```python
from build123d import *

# Parameters (mm, degrees)
SKETCH_1_R          = 20
SKETCH_1_R_2        = 1.6
EXTRUDE_1_DEPTH     = 2.5
SWEEP_1_PROFILE_R   = 5
EXTRUDE_2_DEPTH     = 2.5
SKETCH_10_W         = 23
SKETCH_10_H         = 44.650800955
CUT_EXTRUDE_1_DEPTH = 2
SKETCH_11_R         = 2.5
CUT_EXTRUDE_2_DEPTH = 21.5
FILLET_1_R          = 5


with BuildPart() as part:
    # 草图1 → 凸台-拉伸1 (new body, symmetric)
    with BuildSketch(Plane.XY):
        Circle(SKETCH_1_R)
        with Locations((0, 15)):
            Circle(SKETCH_1_R_2, mode=Mode.SUBTRACT)
        with Locations((15, 0)):
            Circle(SKETCH_1_R_2, mode=Mode.SUBTRACT)
        with Locations((0, -15)):
            Circle(SKETCH_1_R_2, mode=Mode.SUBTRACT)
        with Locations((-15, 0)):
            Circle(SKETCH_1_R_2, mode=Mode.SUBTRACT)
    extrude(amount=EXTRUDE_1_DEPTH, both=True)

    # 扫描1: sweep along a path in 草图4
    with BuildLine(Plane(origin=(0, 0, 0), x_dir=(1, 0, 0), z_dir=(0, 1, 0))) as sweep_1_path:
        Line((0, 0), (0, 60))
    # 扫描1 profile (on start of the path) → 扫描1 (sweep)
    with BuildSketch(Plane(origin=(0, 0, 0), x_dir=(-1, 0, 0), z_dir=(0, 0, -1))):
        Circle(SWEEP_1_PROFILE_R)
    sweep(path=sweep_1_path.line)

    # 草图9 → 凸台-拉伸2 (add, symmetric)
    with BuildSketch(Plane(origin=(0, 0, 0), x_dir=(1, 0, 0), z_dir=(0, 1, 0))):
        with BuildLine():
            Line((13.5, 90), (13.5, 60))
            ThreePointArc((13.5, 60), (0, 46.5), (-13.5, 60))
            Line((-13.5, 60), (-13.5, 90))
            ThreePointArc((-13.5, 90), (0, 103.5), (13.5, 90))
        make_face()
    extrude(amount=EXTRUDE_2_DEPTH, both=True)

    # 草图10 → 切除-拉伸1 (cut)
    with BuildSketch(Plane(origin=(0, 2.5, 0), x_dir=(1, 0, 0), z_dir=(0, 1, 0))):
        with Locations((0, 82.325400478)):
            Rectangle(SKETCH_10_W, SKETCH_10_H)
    extrude(amount=-CUT_EXTRUDE_1_DEPTH, mode=Mode.SUBTRACT)

    # 草图11 → 切除-拉伸2 (cut, through all)
    with BuildSketch(Plane(origin=(0, 0.5, 0), x_dir=(1, 0, 0), z_dir=(0, 1, 0))):
        with Locations((-6.75, 64)):
            Circle(SKETCH_11_R)
        with Locations((6.75, 64)):
            Circle(SKETCH_11_R)
    extrude(amount=-CUT_EXTRUDE_2_DEPTH, mode=Mode.SUBTRACT)

    # 圆角1
    fillet_1_edges = [part.edges().sort_by_distance(p)[0] for p in [
        (5, 0, -2.5),
        (4.330127019, -2.5, -53.606644074),
        (-4.330127019, -2.5, -53.606644074),
        (4.330127019, 2.5, -53.606644074),
        (-4.330127019, 2.5, -53.606644074),
    ]]
    fillet(fillet_1_edges, radius=FILLET_1_R)


solid = part.part
```
Geometry check sheet. Reference: the model listing, model coordinates, mm. A direction names the side the tool comes from. Give positions to 0.01 mm unless a question says otherwise; leave off trailing zeros. Order: outer loops, then holes, each group sorted by start corner. A loop starts at its lowest first (then second) coordinate and runs counter-clockwise, first axis right, second up. Notation, with made-up numbers: (15.5, 17) - (71.5, 17) arc R13 ccw to (71.5, 25) - close; hole circle Ø7 at (36, 3.5). An arc over 180 degrees is marked (long way). Write item = value, one per line. Start each with the question number.
1) Access from +Z, -Z, +X, -X, +Y, -Y to the whole of each face (thin tool, end or side, straight path). Record for faces 5 (the flat face through (0, 0.5, -82)), 6 (the flat face through (-12, 2.5, -68)), 7 (the flat face through (12, 2.5, -68)), 8 (the flat face through (-13.5, 0, -75)), 9 (the flat face through (13.5, 0, -75)).
2) Draft check along Z on faces 1 (the cylindrical face through (6.42, -0.98, -66.48)), 2 (the flat face through (0, 0, 2.5)), 3 (the cylindrical face through (-16.6, 0.07, -0.04)), 4 (the cylindrical face through (-0.297, -0.521, -103.497)). Enter one of: released by +Z, released by -Z, zero draft, split by the parting line, or undercut.
3) Section check C-C (z = -84.5). Enter the section's corners in (x, y).
4) Gauge pin test, flat ends, axial feed: pin 1 Ø3 at (x, z) = (-8, -32) entering from +Y; pin 2 Ø1.5 at (y, z) = (-1, -67.5) entering from +X; pin 3 Ø7.5 at (x, z) = (-10, -83) entering from +Y; pin 4 Ø1.3 at (x, y) = (3, 2) entering from -Z. Record the tip position at first contact, or that the pin passes through.
5) Section check B-B (y = -15). Enter the section's corners in (x, z).
6) Scan lines: L1, parallel to X at y = -0.35, z = -64; L2, parallel to Z at x = 6, y = 0; L3, parallel to Z at x = 6.75, y = -0.4. Record each from-to range of solid material in increasing order.
7) Section check A-A (x = 0). Enter the section's corners in (y, z), then the cut area to 3 significant figures.
Geometry check:
q1.face_5 = -Z, +Y
q1.face_6 = -Z, -X, +Y
q1.face_7 = -Z, +X, +Y
q1.face_8 = -Z, -X, +Y, -Y
q1.face_9 = -Z, +X, +Y, -Y
q2.face_1 = undercut
q2.face_2 = released by +Z
q2.face_3 = zero draft
q2.face_4 = released by -Z
q3.outline = (-13.5, -2.5) - (13.5, -2.5) - (13.5, 2.5) - (11.5, 2.5) - (11.5, 0.5) - (-11.5, 0.5) - (-11.5, 2.5) - (-13.5, 2.5) - close
q4.pin_1 = through
q4.pin_2 = 13.5
q4.pin_3 = 2.5
q4.pin_4 = -60
q5.outline = (-13.23, -2.5) - (-1.6, -2.5) - (-1.6, 2.5) - (-13.23, 2.5) - close; (1.6, -2.5) - (13.23, -2.5) - (13.23, 2.5) - (1.6, 2.5) - close
q6.L1 = -13.5 to -9.25, -4.25 to 4.25, 9.25 to 13.5
q6.L2 = -102.09 to -66.38, -61.62 to -47.91, -4.5 to 2.5
q6.L3 = -101.69 to -66.5, -61.5 to -48.31, -3.69 to 2.5
q7.outline = (-20, -2.5) - (-16.6, -2.5) - (-16.6, 2.5) - (-20, 2.5) - close; (-13.4, -2.5) - (-10, -2.5) arc R5 cw to (-5, -7.5) - (-5, -60) - (-2.5, -60) - (-2.5, -103.5) - (0.5, -103.5) - (0.5, -60) - (5, -60) - (5, -7.5) arc R5 cw to (10, -2.5) - (13.4, -2.5) - (13.4, 2.5) - (-13.4, 2.5) - close; (16.6, -2.5) - (20, -2.5) - (20, 2.5) - (16.6, 2.5) - close
q7.area = 884 mm2
